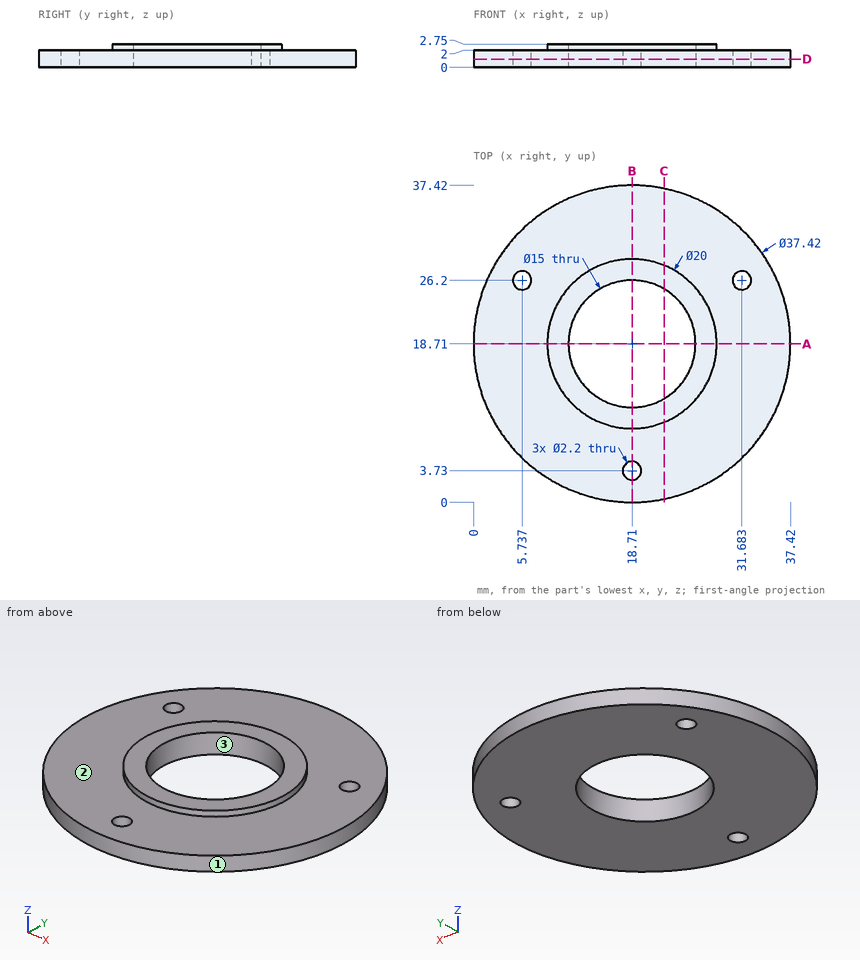
Input: dimensioned drawing with shaded views. Units: mm. Origin: part minimum x, y, z. Round coordinates to 2 decimals unless told otherwise and drop trailing zeros. Order: outer loops, then holes, each group sorted by start corner. A loop starts at its lowest first (then second) coordinate and runs counter-clockwise, first axis right, second up. Notation, with made-up numbers: (30, 15) -> (50, 15) arc R17 cw to (50, 34) -> close; hole circle Ø5 at (25, 47). An arc over 180 degrees is marked (long way). Put each result on its own line as item: value. Start each with the question number.
Q1. Section C-C on x = 22.5. Return the cut outline in (y, z), and give its area (3 significant figures).
Q2. First-contact query: pin 1 (1 mm diameter, centred on y = 27.5, z = 2, fed in from +X). Flat tip, straight axial feed; report the tip coordinate or a pass-through.
Q3. Section D-D on z = 0.95. Return the cut outline in (x, y).
Q4. Line query: probe 1 along Y at (x, z) = (18.71, 1.7); probe 2 along Z at (x, y) = (33.5, 18.5); probe 3 along X at (y, z) = (16, 2.3). Output: solid intervals per line, ascending.
Q5. Pull-direction query (Y, two-part tool) for the marked faces 1, 2 and 3; classes: +Y half, -Y half, draft (parallel to the pull), parting line (faces both ways), or undercut.
Q6. Section A-A on y = 18.71. Return the cut outline in (x, z).
Q7. Section B-B on x = 18.71. Return the cut outline in (y, z), and give its area (3 significant figures).
Ans:
1. outline: (0.39, 0) -> (12.24, 0) -> (12.24, 2.75) -> (9.46, 2.75) -> (9.46, 2) -> (0.39, 2) -> close; (25.18, 0) -> (37.03, 0) -> (37.03, 2) -> (27.96, 2) -> (27.96, 2.75) -> (25.18, 2.75) -> close
1. area: 51.6 mm2
2. pin 1: stops at x = 35.48
3. outline: circle Ø37.42 at (18.71, 18.71); hole circle Ø2.2 at (5.74, 26.2); hole circle Ø15 at (18.71, 18.71); hole circle Ø2.2 at (18.71, 3.73); hole circle Ø2.2 at (31.68, 26.2)
4. probe 1: y = 0 to 2.63, 4.83 to 11.21, 26.21 to 37.42
4. probe 2: z = 0 to 2
4. probe 3: x = 9.08 to 11.72, 25.7 to 28.34
5. face 1: parting line
5. face 2: draft
5. face 3: undercut
6. outline: (0, 0) -> (11.21, 0) -> (11.21, 2.75) -> (8.71, 2.75) -> (8.71, 2) -> (0, 2) -> close; (26.21, 0) -> (37.42, 0) -> (37.42, 2) -> (28.71, 2) -> (28.71, 2.75) -> (26.21, 2.75) -> close
7. outline: (0, 0) -> (2.63, 0) -> (2.63, 2) -> (0, 2) -> close; (4.83, 0) -> (11.21, 0) -> (11.21, 2.75) -> (8.71, 2.75) -> (8.71, 2) -> (4.83, 2) -> close; (26.21, 0) -> (37.42, 0) -> (37.42, 2) -> (28.71, 2) -> (28.71, 2.75) -> (26.21, 2.75) -> close
7. area: 44.2 mm2
